Model file for the job. Use its own axes, mm. A direction names the side the tool comes from. Give positions to 0.01 mm unless a question says otherwise; leave off trailing zeros. Loops run counter-clockwise (first coordinate to the right, second up) from the corner with the lowest first, then second, coordinate; pieces in that order, holes last. Notation, with made-up numbers: (-31.75, 73) - (-13.75, 73) arc R25 cw to (-13.75, 112) - close; hole circle Ø8 at (10, 11.25). An arc over 180 degrees is marked (long way). Answer as CSV lines item,"result". Start each with the question number.
Item 1: Saw through at B-B on x = -26. Give the cut face in (y, z), plus the area to 3 significant figures.
Item 2: Pin check, flat tips, straight feed: pin 1 (2 mm diameter, centred on x = -19.5, y = -5, fed in from +Z); pin 2 (3 mm diameter, centred on y = -10.5, z = -12, fed in from +X); pin 3 (1.5 mm diameter, centred on x = -8, y = -3.5, fed in from +Z). Stop position of each tip, or through.
Item 3: Pull direction Z, two halves, no side cores. Call faces 4 (the flat face through (-40.413, -5.916, -34.278)), 5 (the cylindrical face through (-50, -6, 0)): pulls with the +Z half, pulls with the -Z half, needs draft (parallel to the pull), parting line crosses it, or undercut.
Item 4: Saw through at D-D on y = -4.5. State how many separate pieces and enclosed holes the cut face has, plus the area to 3 significant figures.
Item 5: Saw through at C-C on z = -27.5. Give the cut face in (x, y).
Item 6: Saw through at A-A on x = 0. Give the cut face in (y, z).
Item 7: Drill centre lines: L1, parallel to Z at x = 0, y = -6.5; L2, parallel to X at y = -1.5, z = 16; L3, parallel to X at y = -4.25, z = -33. Where is each one in solid material? Low to high. Write a range as from..to.
Item 8: Tool access for faces 1 (the flat face through (49.81, -5.92, 17.83)), 2 (the flat face through (-9.465, -5.916, -52.056)), 3 (the cylindrical face through (5.042, -5.916, 8.636)): list every direction of +Z, -Z, +X, -X, +Y, -Y with a clear straight run to the whole face (end or side of a thin tool).
from build123d import *

# Parameters (mm, degrees)
F1_DEPTH = 1.2
F2_SCALE = 10
F4_D     = 3


with BuildPart() as f1:
    # F0 (on Front) → F1 (new body)
    with BuildSketch(Plane.XZ):
        with BuildLine():
            Line((-3.7659962211, 1.3480624848), (-4.7074952763, 1.685078106))
            ThreePointArc((-4.7074952763, 1.685078106), (-5, 0), (-4.7074952763, -1.685078106))
            Line((-4.7074952763, -1.685078106), (-3.7659962211, -1.3480624848))
            ThreePointArc((-3.7659962211, -1.3480624848), (-4, 0), (-3.7659962211, 1.3480624848))
        make_face()
        with BuildLine():
            Line((-3.0504544683, 2.5874171556), (-3.8130680853, 3.2342714445))
            Line((-3.8130680853, 3.2342714445), (-4.2631397208, 3.6160254038))
            ThreePointArc((-4.2631397208, 3.6160254038), (-5.6291651246, 3.25), (-5.2631397208, 1.8839745962))
            Line((-5.2631397208, 1.8839745962), (-4.7074952763, 1.685078106))
            Line((-4.7074952763, 1.685078106), (-3.7659962211, 1.3480624848))
            Line((-3.7659962211, 1.3480624848), (-0.9414990553, 0.3370156212))
            ThreePointArc((-0.9414990553, 0.3370156212), (-0.8660254038, 0.5), (-0.7626136171, 0.6468542889))
            Line((-0.7626136171, 0.6468542889), (-3.0504544683, 2.5874171556))
        make_face()
        with BuildLine():
            Line((-0.7155417528, 3.9354796404), (-0.894427191, 4.9193495505))
            ThreePointArc((-0.894427191, 4.9193495505), (-2.5, 4.3301270189), (-3.8130680853, 3.2342714445))
            Line((-3.8130680853, 3.2342714445), (-3.0504544683, 2.5874171556))
            ThreePointArc((-3.0504544683, 2.5874171556), (-2, 3.4641016151), (-0.7155417528, 3.9354796404))
        make_face()
        with BuildLine():
            Line((-1, 5.5), (-0.894427191, 4.9193495505))
            Line((-0.894427191, 4.9193495505), (-0.7155417528, 3.9354796404))
            Line((-0.7155417528, 3.9354796404), (-0.1788854382, 0.9838699101))
            ThreePointArc((-0.1788854382, 0.9838699101), (0, 1), (0.1788854382, 0.9838699101))
            Line((0.1788854382, 0.9838699101), (0.7155417528, 3.9354796404))
            Line((0.7155417528, 3.9354796404), (0.894427191, 4.9193495505))
            Line((0.894427191, 4.9193495505), (1, 5.5))
            ThreePointArc((1, 5.5), (0, 6.5), (-1, 5.5))
        make_face()
        with BuildLine():
            ThreePointArc((3.8130680853, 3.2342714445), (2.5, 4.3301270189), (0.894427191, 4.9193495505))
            Line((0.894427191, 4.9193495505), (0.7155417528, 3.9354796404))
            ThreePointArc((0.7155417528, 3.9354796404), (2, 3.4641016151), (3.0504544683, 2.5874171556))
            Line((3.0504544683, 2.5874171556), (3.8130680853, 3.2342714445))
        make_face()
        with BuildLine():
            Line((3.0504544683, 2.5874171556), (0.7626136171, 0.6468542889))
            ThreePointArc((0.7626136171, 0.6468542889), (0.8660254038, 0.5), (0.9414990553, 0.3370156212))
            Line((0.9414990553, 0.3370156212), (3.7659962211, 1.3480624848))
            Line((3.7659962211, 1.3480624848), (4.7074952763, 1.685078106))
            Line((4.7074952763, 1.685078106), (5.2631397208, 1.8839745962))
            ThreePointArc((5.2631397208, 1.8839745962), (5.6291651246, 3.25), (4.2631397208, 3.6160254038))
            Line((4.2631397208, 3.6160254038), (3.8130680853, 3.2342714445))
            Line((3.8130680853, 3.2342714445), (3.0504544683, 2.5874171556))
        make_face()
        with BuildLine():
            Line((4.7074952763, 1.685078106), (3.7659962211, 1.3480624848))
            ThreePointArc((3.7659962211, 1.3480624848), (4, 0), (3.7659962211, -1.3480624848))
            Line((3.7659962211, -1.3480624848), (4.7074952763, -1.685078106))
            ThreePointArc((4.7074952763, -1.685078106), (5, 0), (4.7074952763, 1.685078106))
        make_face()
        with BuildLine():
            Line((3.7659962211, -1.3480624848), (0.9414990553, -0.3370156212))
            ThreePointArc((0.9414990553, -0.3370156212), (0.8660254038, -0.5), (0.7626136171, -0.6468542889))
            Line((0.7626136171, -0.6468542889), (3.0504544683, -2.5874171556))
            Line((3.0504544683, -2.5874171556), (3.8130680853, -3.2342714445))
            Line((3.8130680853, -3.2342714445), (4.2631397208, -3.6160254038))
            ThreePointArc((4.2631397208, -3.6160254038), (5.6291651246, -3.25), (5.2631397208, -1.8839745962))
            Line((5.2631397208, -1.8839745962), (4.7074952763, -1.685078106))
            Line((4.7074952763, -1.685078106), (3.7659962211, -1.3480624848))
        make_face()
        with BuildLine():
            ThreePointArc((3.0504544683, -2.5874171556), (2, -3.4641016151), (0.7155417528, -3.9354796404))
            Line((0.7155417528, -3.9354796404), (0.894427191, -4.9193495505))
            ThreePointArc((0.894427191, -4.9193495505), (2.5, -4.3301270189), (3.8130680853, -3.2342714445))
            Line((3.8130680853, -3.2342714445), (3.0504544683, -2.5874171556))
        make_face()
        with BuildLine():
            ThreePointArc((0.1788854382, -0.9838699101), (0, -1), (-0.1788854382, -0.9838699101))
            Line((-0.1788854382, -0.9838699101), (-0.7155417528, -3.9354796404))
            Line((-0.7155417528, -3.9354796404), (-0.894427191, -4.9193495505))
            Line((-0.894427191, -4.9193495505), (-1, -5.5))
            ThreePointArc((-1, -5.5), (0, -6.5), (1, -5.5))
            Line((1, -5.5), (0.894427191, -4.9193495505))
            Line((0.894427191, -4.9193495505), (0.7155417528, -3.9354796404))
            Line((0.7155417528, -3.9354796404), (0.1788854382, -0.9838699101))
        make_face()
        with BuildLine():
            ThreePointArc((-0.7626136171, -0.6468542889), (-0.8660254038, -0.5), (-0.9414990553, -0.3370156212))
            Line((-0.9414990553, -0.3370156212), (-3.7659962211, -1.3480624848))
            Line((-3.7659962211, -1.3480624848), (-4.7074952763, -1.685078106))
            Line((-4.7074952763, -1.685078106), (-5.2631397208, -1.8839745962))
            ThreePointArc((-5.2631397208, -1.8839745962), (-5.6291651246, -3.25), (-4.2631397208, -3.6160254038))
            Line((-4.2631397208, -3.6160254038), (-3.8130680853, -3.2342714445))
            Line((-3.8130680853, -3.2342714445), (-3.0504544683, -2.5874171556))
            Line((-3.0504544683, -2.5874171556), (-0.7626136171, -0.6468542889))
        make_face()
        with BuildLine():
            ThreePointArc((0.1788854382, 0.9838699101), (0, 1), (-0.1788854382, 0.9838699101))
            ThreePointArc((-0.1788854382, 0.9838699101), (-0.5, 0.8660254038), (-0.7626136171, 0.6468542889))
            ThreePointArc((-0.7626136171, 0.6468542889), (-0.8660254038, 0.5), (-0.9414990553, 0.3370156212))
            ThreePointArc((-0.9414990553, 0.3370156212), (-1, 0), (-0.9414990553, -0.3370156212))
            ThreePointArc((-0.9414990553, -0.3370156212), (-0.8660254038, -0.5), (-0.7626136171, -0.6468542889))
            ThreePointArc((-0.7626136171, -0.6468542889), (-0.5, -0.8660254038), (-0.1788854382, -0.9838699101))
            ThreePointArc((-0.1788854382, -0.9838699101), (0, -1), (0.1788854382, -0.9838699101))
            ThreePointArc((0.1788854382, -0.9838699101), (0.5, -0.8660254038), (0.7626136171, -0.6468542889))
            ThreePointArc((0.7626136171, -0.6468542889), (0.8660254038, -0.5), (0.9414990553, -0.3370156212))
            ThreePointArc((0.9414990553, -0.3370156212), (0.9852662217, -0.1710276947), (1, 0))
            ThreePointArc((1, 0), (0.9852662217, 0.1710276947), (0.9414990553, 0.3370156212))
            ThreePointArc((0.9414990553, 0.3370156212), (0.8660254038, 0.5), (0.7626136171, 0.6468542889))
            ThreePointArc((0.7626136171, 0.6468542889), (0.5, 0.8660254038), (0.1788854382, 0.9838699101))
        make_face()
        with BuildLine():
            ThreePointArc((-0.7155417528, -3.9354796404), (-2, -3.4641016151), (-3.0504544683, -2.5874171556))
            Line((-3.0504544683, -2.5874171556), (-3.8130680853, -3.2342714445))
            ThreePointArc((-3.8130680853, -3.2342714445), (-2.5, -4.3301270189), (-0.894427191, -4.9193495505))
            Line((-0.894427191, -4.9193495505), (-0.7155417528, -3.9354796404))
        make_face()
    extrude(amount=F1_DEPTH)


with BuildPart() as f1_1:
    # F2: moved
    add(f1.part.scale(F2_SCALE))

    # F4 (through all)
    with Locations(Plane(origin=(0, 0, 0), x_dir=(1, 0, 0), z_dir=(0, 1, 0))):
        with Locations((0, 0)):
            Hole(F4_D / 2)


solid = f1_1.part
Responses:
1,outline,"(-12, -42.71) - (0, -42.71) - (0, -30.4) - (-12, -30.4) - close; (-12, -22.05) - (0, -22.05) - (0, -9.31) - (-12, -9.31) - close; (-12, 9.31) - (0, 9.31) - (0, 22.05) - (-12, 22.05) - close; (-12, 30.4) - (0, 30.4) - (0, 42.71) - (-12, 42.71) - close"
1,area,"601 mm2"
2,pin 1,"z = 46.45"
2,pin 2,"x = 48.89"
2,pin 3,"z = 61.89"
3,face 4,"pulls with the -Z half"
3,face 5,"undercut"
4,separate pieces,"1"
4,enclosed holes,"7"
4,area,"6,300 mm2"
5,outline,"(-57.63, -12) - (-29.05, -12) - (-29.05, 0) - (-57.63, 0) - close; (-5, -12) - (5, -12) - (5, 0) - (-5, 0) - close; (29.05, -12) - (57.63, -12) - (57.63, 0) - (29.05, 0) - close"
6,outline,"(-12, -65) - (0, -65) - (0, -1.5) - (-12, -1.5) - close; (-12, 1.5) - (0, 1.5) - (0, 65) - (-12, 65) - close"
7,L1,"-65..-1.5, 1.5..65"
7,L2,"-47.37..-18.86, -2.91..2.91, 18.86..47.37"
7,L3,"-55.98..-38.91, -37.56..-22.61, -6..6, 22.61..37.56, 38.91..55.98"
8,face 1,"+X, +Y, -Y"
8,face 2,"-X, +Y, -Y"
8,face 3,"+Y, -Y"
